Source: CAD feature listing. Evaluate the final solid. Frame: model axes, mm. A direction names the side the tool comes from. Coordinates: 2 decimals unless noted, no trailing zeros. Write each loop counter-clockwise with the first axis right and the second up, starting at its lowest first coordinate (ties: lowest second). Pieces come first, ordered by that corner, then holes. Notation, with made-up numbers: (-37, -4) -> (0, -4) arc R31 cw to (0, 25) -> close; hole circle Ø7 at (57.5, 31.25). An arc over 180 degrees is marked (long way). Write item = value, one per line.
from build123d import *

# Parameters (mm, degrees)
F1_DEPTH       = 30
F3_D           = 12.6
F3_CBORE_D     = 19.25
F3_CBORE_DEPTH = 12
F5_DEPTH       = 20
F7_DEPTH       = 10
F9_DEPTH       = 51.5
F10_R          = 2


with BuildPart() as f1:
    # F0 (on Front) → F1 (new body)
    with BuildSketch(Plane.XZ):
        with BuildLine():
            Line((0, -30), (0, 0))
            Line((0, 0), (30, 30))
            Line((30, 30), (50, 30))
            ThreePointArc((50, 30), (57.0710678119, 32.9289321881), (60, 40))
            Line((60, 40), (60, 50))
            ThreePointArc((60, 50), (57.0710678119, 57.0710678119), (50, 60))
            Line((50, 60), (-40, 60))
            ThreePointArc((-40, 60), (-47.0710678119, 57.0710678119), (-50, 50))
            Line((-50, 50), (-50, -30))
            ThreePointArc((-50, -30), (-47.0710678119, -37.0710678119), (-40, -40))
            Line((-40, -40), (-10, -40))
            ThreePointArc((-10, -40), (-2.9289321881, -37.0710678119), (0, -30))
        make_face()
    extrude(amount=F1_DEPTH)

    # F3 (through all)
    with Locations(Plane.XZ.offset(30)):
        with Locations((45, 45)):
            CounterBoreHole(F3_D / 2, F3_CBORE_D / 2, F3_CBORE_DEPTH)

    # F4 (on face) → F5 (cut)
    with BuildSketch(Plane.XZ.offset(30)):
        with BuildLine():
            Line((-5.0000011261, -30), (-5.0000011261, 0))
            Line((-5.0000011261, 0), (-5.0000011261, 50))
            ThreePointArc((-5.0000011261, 50), (-6.4644668903, 53.5355331097), (-10, 54.9999988739))
            Line((-10, 54.9999988739), (-40, 54.9999988739))
            ThreePointArc((-40, 54.9999988739), (-43.5355331097, 53.5355331097), (-44.9999988739, 50))
            Line((-44.9999988739, 50), (-44.9999988739, -30))
            ThreePointArc((-44.9999988739, -30), (-43.5355331097, -33.5355331097), (-40, -34.9999988739))
            Line((-40, -34.9999988739), (-10, -34.9999988739))
            ThreePointArc((-10, -34.9999988739), (-6.4644668903, -33.5355331097), (-5.0000011261, -30))
        make_face()
    extrude(amount=-F5_DEPTH, mode=Mode.SUBTRACT)

    # F6 (on face) → F7 (join)
    with BuildSketch(Plane.XZ.offset(10)):
        with BuildLine():
            ThreePointArc((-35.0377668691, -10), (-25.0377668691, -20), (-15.0377668691, -10))
            Line((-15.0377668691, -10), (-15.0377668691, 25))
            ThreePointArc((-15.0377668691, 25), (-25.0377668691, 35), (-35.0377668691, 25))
            Line((-35.0377668691, 25), (-35.0377668691, -10))
        make_face()
    extrude(amount=F7_DEPTH)

    # F8 (on face) → F9 (cut, symmetric)
    with BuildSketch(Plane.XZ.offset(20)):
        with BuildLine():
            ThreePointArc((-30.0377668691, -10), (-25.0377668691, -15), (-20.0377668691, -10))
            Line((-20.0377668691, -10), (-20.0377668691, 25))
            ThreePointArc((-20.0377668691, 25), (-25.0377668691, 30), (-30.0377668691, 25))
            Line((-30.0377668691, 25), (-30.0377668691, -10))
        make_face()
    extrude(amount=F9_DEPTH, both=True, mode=Mode.SUBTRACT)

    # F10
    f10_edges = [f1.edges().sort_by_distance(p)[0] for p in [
        (-5.000001, -10, 10),
        (-6.464467, -10, -33.535533),
        (-6.464467, -10, 53.535533),
        (-25, -10, -34.999999),
        (-25, -10, 54.999999),
        (-43.535533, -10, -33.535533),
        (-43.535533, -10, 53.535533),
        (-44.999999, -10, 10),
        (-35.037767, -10, 7.5),
        (-25.037767, -10, -20),
        (-15.037767, -10, 7.5),
        (-25.037767, -10, 35),
    ]]
    fillet(f10_edges, radius=F10_R)


solid = f1.part
1) First-contact query: pin 1 Ø8 at (x, y) = (-3.5, -17) entering from -Z; pin 2 Ø10 at (x, y) = (-1, -3.5) entering from -Z; pin 3 Ø6 at (y, z) = (-11, 6) entering from +X. Flat tips, straight axial feed; report the tip coordinate or a pass-through.
Answer block:
pin_1 = -39.68
pin_2 = -39.17
pin_3 = 9
2) Cut plane B-B, the plane z = 20. Output: boundary loops of the cut face in (x, y).
Answer block:
outline = (-50, -30) -> (-45, -30) -> (-45, -12) arc R2 cw to (-43, -10) -> (-37.04, -10) arc R2 cw to (-35.04, -12) -> (-35.04, -20) -> (-30.04, -20) -> (-30.04, 0) -> (-50, 0) -> close; (-20.04, -20) -> (-15.04, -20) -> (-15.04, -12) arc R2 cw to (-13.04, -10) -> (-7, -10) arc R2 cw to (-5, -12) -> (-5, -30) -> (20, -30) -> (20, 0) -> (-20.04, 0) -> close
3) Pull-direction query (Z, two-part tool) for faces 1 (the flat face through (-45, -21, 11)), 2 (the cylindrical face through (57.15, -14.79, 56.99)), 3 (the flat face through (0, -15, -15)); classes: +Z half, -Z half, draft (parallel to the pull), parting line (faces both ways), or undercut.
Answer block:
face_1 = undercut
face_2 = +Z half
face_3 = draft
4) Cut plane C-C, the plane y = -4.25. Output: boundary loops of the cut face in (x, z).
Answer block:
outline = (-50, -30) arc R10 ccw to (-40, -40) -> (-10, -40) arc R10 ccw to (0, -30) -> (0, 0) -> (30, 30) -> (50, 30) arc R10 ccw to (60, 40) -> (60, 50) arc R10 ccw to (50, 60) -> (-40, 60) arc R10 ccw to (-50, 50) -> close; hole (-30.04, -10) arc R5 ccw to (-20.04, -10) -> (-20.04, 25) arc R5 ccw to (-30.04, 25) -> close; hole circle Ø12.6 at (45, 45)
5) Reachability of faces 4 (the cylindrical face through (-25, -16, -20)), 5 (the cylindrical face through (-46.99, -14.79, 57.15)), 6 (the flat face through (-30.038, -10, 8)) from +Z, -Z, +X, -X, +Y, -Y: full face, straight path, thin tool, end or side. Return the list, or none.
Answer block:
face_4 = -Y
face_5 = +Z, -X, +Y, -Y
face_6 = +Y, -Y
6) Cut plane A-A, the plane y = -13.5. Give the number of separate pieces and of enclosed holes in the cut face, and give its area (3 significant figures).
Answer block:
separate_pieces = 2
enclosed_holes = 3
area = 4,030 mm2
7) Material intervals for probe 1 along X at (y, z) = (-16, -14); probe 2 along X at (y, z) = (-25, 48.5); probe 3 along Z at (x, y) = (-18.5, -19), sorted ascending. Write a range as [from, to].
Answer block:
probe_1 = [-50, -45], [-34.2, -28.04], [-22.04, -15.87], [-5, 0]
probe_2 = [-50, -45], [-5, 36.03], [53.97, 60]
probe_3 = [-40, -35], [-17.57, 32.57], [55, 60]
8) Cut plane D-D, the plane z = 5. Output: boundary loops of the cut face in (x, y).
Answer block:
outline = (-50, -30) -> (-45, -30) -> (-45, -12) arc R2 cw to (-43, -10) -> (-37.04, -10) arc R2 cw to (-35.04, -12) -> (-35.04, -20) -> (-30.04, -20) -> (-30.04, 0) -> (-50, 0) -> close; (-20.04, -20) -> (-15.04, -20) -> (-15.04, -12) arc R2 cw to (-13.04, -10) -> (-7, -10) arc R2 cw to (-5, -12) -> (-5, -30) -> (5, -30) -> (5, 0) -> (-20.04, 0) -> close
